from build123d import *

# Parameters (mm, degrees)
F0_W     = 40
F0_H     = 59
F1_DEPTH = 25
F2_R     = 3


with BuildPart() as f1:
    # F0 (on Top) → F1 (new body)
    with BuildSketch(Plane.XY):
        Rectangle(F0_W, F0_H)
        with BuildLine():
            ThreePointArc((-13, 23.45), (-14.0960155108, 26.0960155108), (-11.45, 25))
            Line((-11.45, 25), (11.45, 25))
            ThreePointArc((11.45, 25), (13, 26.55), (14.55, 25))
            ThreePointArc((14.55, 25), (14.0960155108, 23.9039844892), (13, 23.45))
            Line((13, 23.45), (13, -23.45))
            ThreePointArc((13, -23.45), (14.0960155108, -23.9039844892), (14.55, -25))
            ThreePointArc((14.55, -25), (13, -26.55), (11.45, -25))
            Line((11.45, -25), (-11.5, -25))
            ThreePointArc((-11.5, -25), (-14.0606601718, -26.0606601718), (-13, -23.5))
            Line((-13, -23.5), (-13, 23.45))
        make_face(mode=Mode.SUBTRACT)
        with BuildLine():
            Line((11.45, 25), (-11.45, 25))
            ThreePointArc((-11.45, 25), (-11.9039844892, 23.9039844892), (-13, 23.45))
            Line((-13, 23.45), (-13, -23.5))
            ThreePointArc((-13, -23.5), (-11.9393398282, -23.9393398282), (-11.5, -25))
            Line((-11.5, -25), (11.45, -25))
            ThreePointArc((11.45, -25), (11.9039844892, -23.9039844892), (13, -23.45))
            Line((13, -23.45), (13, 23.45))
            ThreePointArc((13, 23.45), (11.9039844892, 23.9039844892), (11.45, 25))
        make_face()
    extrude(amount=F1_DEPTH)

    # F2
    f2_edges = [f1.edges().sort_by_distance(p)[0] for p in [
        (-20, 29.5, 12.5),
        (20, 29.5, 12.5),
        (20, -29.5, 12.5),
        (-20, -29.5, 12.5),
    ]]
    fillet(f2_edges, radius=F2_R)


solid = f1.part
The model under review builds one solid part; all positions refer to its coordinate system, in mm. Coordinates: 2 decimals unless noted, no trailing zeros. Write each loop counter-clockwise with the first axis right and the second up, starting at its lowest first coordinate (ties: lowest second). Pieces come first, ordered by that corner, then holes. Notation, with made-up numbers: M 33,69 L 77,69 A16 cw 77,85 Z; hole C 72,24.5 d4. An arc over 180 degrees is marked long. Put each result on its own line as item: value.
1) Add section A-A on z = 16.75. Give the boundary of the cut face in (x, y), then the cut area to 3 significant figures.
Computed:
outline: M -20,-26.5 A3 ccw -17,-29.5 L 17,-29.5 A3 ccw 20,-26.5 L 20,26.5 A3 ccw 17,29.5 L -17,29.5 A3 ccw -20,26.5 Z; hole C -13,25 d3.1; hole C -13,-25 d3; hole C 13,-25 d3.1; hole C 13,25 d3.1
area: 2,320 mm2
2) Clearance check with a flat-ended pin moving along its axis: pin 1 Ø1 at (x, y) = (-1, -2) entering from -Z. State where the tip first meets the part, or that it passes through.
Computed:
pin 1: stops at z = 0
3) Wall thickness on probe 1 along X at (y, z) = (-25, 15); probe 2 along Y at (x, z) = (-13, 9.5); probe 3 along X at (y, z) = (-26, 5.75): over which ranges is each line inside the solid? List them lowest first. Write a range as [from, to].
Computed:
probe 1: x = [-20, -14.5], [-11.5, 11.45], [14.55, 20]
probe 2: y = [-29.5, -26.5], [-23.5, 23.45], [26.55, 29.5]
probe 3: x = [-20, -14.12], [-11.88, 11.82], [14.18, 20]
